Design review of the part shown in the three views and the two pictorial views. Dimensions are in mm from the part's minimum x, y and z. A direction names the side the tool comes from. Round coordinates to 2 decimals unless told otherwise and drop trailing zeros. Loops run counter-clockwise (first coordinate to the right, second up) from the corner with the lowest first, then second, coordinate; pieces in that order, holes last.
1) Tool access review of the marked faces 5 and 6: name each direction out of +Z, -Z, +X, -X, +Y, -Y from which nothing blocks a thin tool from reaching the whole face with its end or side.
2) Wall thickness on L1, parallel to Z at x = 6, y = 1.85; L2, parallel to X at y = 1.2, z = 15; L3, parallel to Y at x = 3.75, z = 17: over which ranges is each line inside the solid? List them lowest first.
3) Take a section at C-C (x = 4). State the section outline as (y, z) points.
4) Take a section at A-A (y = 0.8). State the section outline as (x, z) points.
5) Take a section at B-B (z = 8.8). State the section outline as (x, y) points.
6) Take a section at D-D (y = 2.1). State the section outline as (x, z) points.
7) Insertion check: pin 1 (0.7 mm diameter, centred on x = 4, y = 1.5, fed in from -Z); pin 2 (3 mm diameter, centred on x = 2.5, z = 8.5, fed in from +Y). Each pin has a flat end and moves straight along its axis. Give the tip position at first contact, or say it passes through.
8) Mouldability with a two-part tool opening along Z and no side actions: class the marked faces 1, 2, 3 and 4 as pulls with the +Z half, pulls with the -Z half, needs draft (parallel to the pull), parting line crosses it, or undercut.
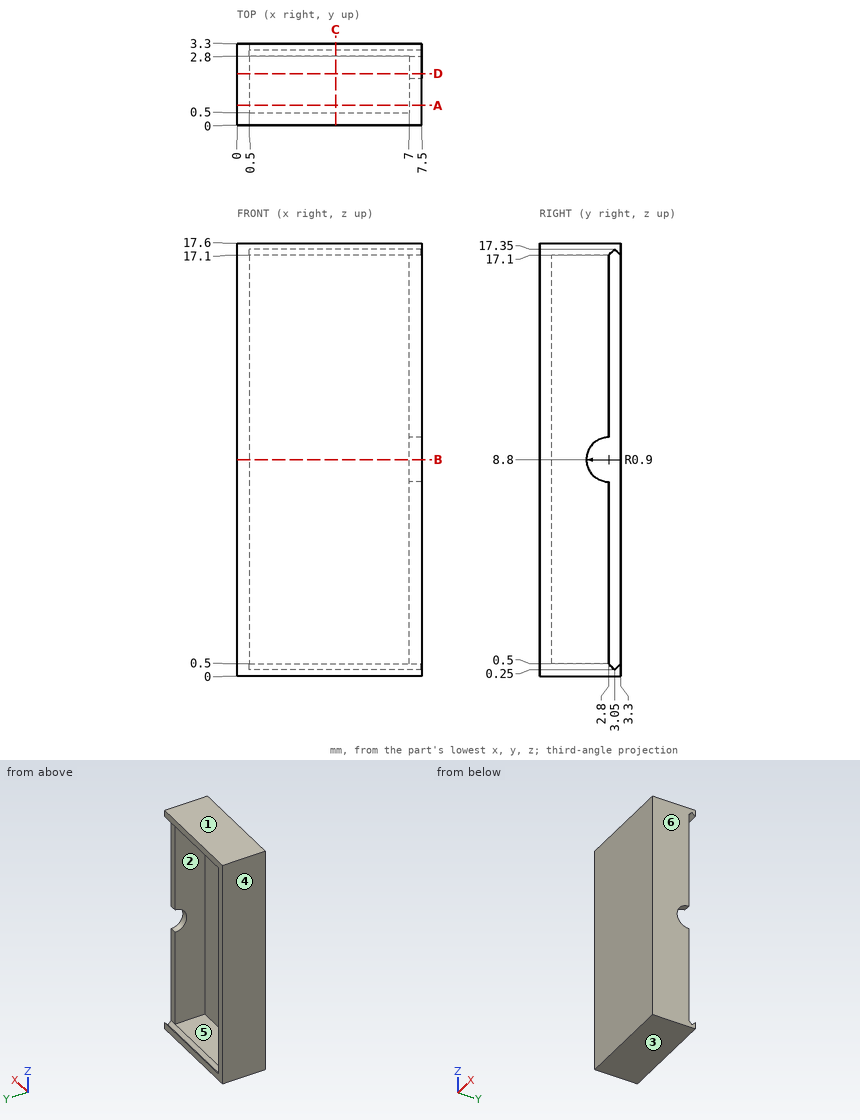
Response:
1. face 5: +Y
1. face 6: +Z, -Z, +X, +Y, -Y
2. L1: z = 0 to 0.5, 17.1 to 17.6
2. L2: x = 0 to 0.5, 7 to 7.5
2. L3: y = 0 to 0.5
3. outline: (0, 0) - (3.3, 0) - (3.3, 0.5) - (3.05, 0.25) - (2.8, 0.5) - (0.5, 0.5) - (0.5, 17.1) - (2.8, 17.1) - (3.05, 17.35) - (3.3, 17.1) - (3.3, 17.6) - (0, 17.6) - close
4. outline: (0, 0) - (7.5, 0) - (7.5, 17.6) - (0, 17.6) - close; hole (0.5, 0.5) - (7, 0.5) - (7, 17.1) - (0.5, 17.1) - close
5. outline: (0, 0) - (7.5, 0) - (7.5, 1.9) - (7, 1.9) - (7, 0.5) - (0.5, 0.5) - (0.5, 3.3) - (0, 3.3) - close
6. outline: (0, 0) - (7.5, 0) - (7.5, 8.23) - (7, 8.23) - (7, 0.5) - (0.5, 0.5) - (0.5, 17.1) - (7, 17.1) - (7, 9.37) - (7.5, 9.37) - (7.5, 17.6) - (0, 17.6) - close
7. pin 1: stops at z = 0
7. pin 2: stops at y = 0.5
8. face 1: pulls with the +Z half
8. face 2: undercut
8. face 3: pulls with the -Z half
8. face 4: needs draft
